Verification items for this drawing (mm, ordinates from the low corner). Coordinates: 2 decimals unless noted, no trailing zeros. Order: outer loops, then holes, each group sorted by start corner. A loop starts at its lowest first (then second) coordinate and runs counter-clockwise, first axis right, second up.
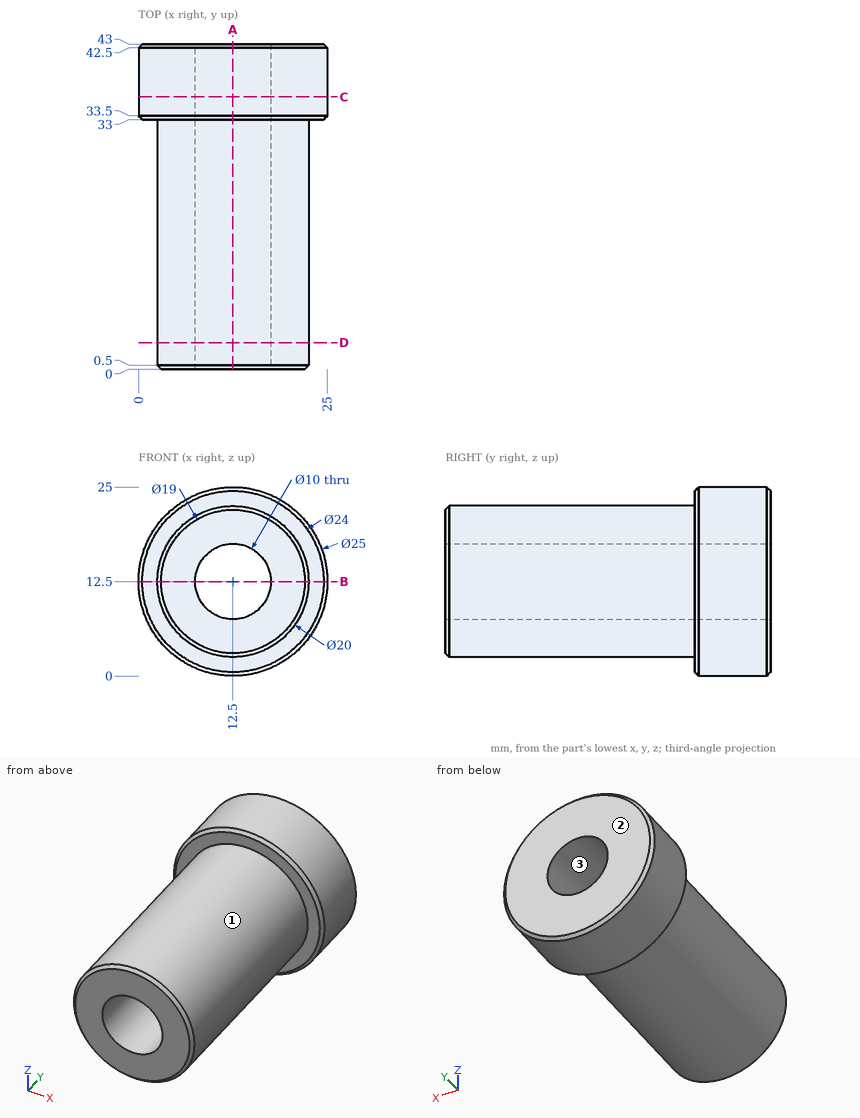
(1) Go/stop test with flat-tipped pins: P1, Ø10, axis at y = 32, z = 4, coming from the -X side; P2, Ø12, axis at x = 5.5, y = 37, coming from the -Z side; P3, Ø8, axis at x = 13.5, y = 24, coming from the +Z side. Record where each tip stops, or that it passes through.
Filled in:
P1: stops at x = 0.57
P2: stops at z = 0.04
P3: stops at z = 22.5
(2) Thickness scan on probe 1 along Z at (x, y) = (12.5, 24); probe 2 along X at (y, z) = (10, 9.25). Record the ranges inside material, lowest first.
Filled in:
probe 1: z = 2.5 to 7.5, 17.5 to 22.5
probe 2: x = 3.04 to 8.7, 16.3 to 21.96
(3) Cross-section at B-B (z = 12.5). Enter the section's corners in (x, y), and give its area (3 significant figures).
Filled in:
outline: (0, 33.5) - (0.5, 33) - (2.5, 33) - (2.5, 0.5) - (3, 0) - (7.5, 0) - (7.5, 43) - (0.5, 43) - (0, 42.5) - close; (17.5, 0) - (22, 0) - (22.5, 0.5) - (22.5, 33) - (24.5, 33) - (25, 33.5) - (25, 42.5) - (24.5, 43) - (17.5, 43) - close
area: 479 mm2
(4) Release check for a two-part mould opening along Z. For the marked faces 1, 2 and 3 record: +Z half, -Z half, draft (parallel to the pull), parting line (faces both ways), or undercut.
Filled in:
face 1: parting line
face 2: draft
face 3: undercut
(5) Cross-section at A-A (x = 12.5). Enter the section's corners in (y, z), and give its area (3 significant figures).
Filled in:
outline: (0, 3) - (0.5, 2.5) - (33, 2.5) - (33, 0.5) - (33.5, 0) - (42.5, 0) - (43, 0.5) - (43, 7.5) - (0, 7.5) - close; (0, 17.5) - (43, 17.5) - (43, 24.5) - (42.5, 25) - (33.5, 25) - (33, 24.5) - (33, 22.5) - (0.5, 22.5) - (0, 22) - close
area: 479 mm2
(6) Cross-section at D-D (y = 3.5). Enter the section's corners in (x, z), and give its area (3 significant figures).
Filled in:
outline: circle Ø20 at (12.5, 12.5); hole circle Ø10 at (12.5, 12.5)
area: 236 mm2
(7) Cross-section at C-C (y = 36). Enter the section's corners in (x, z).
Filled in:
outline: circle Ø25 at (12.5, 12.5); hole circle Ø10 at (12.5, 12.5)
